Can you work these out from the model? Positions are in its coordinate system, mm. Face numbers are marked on the shaded views. A direction names the side the tool comes from. Round coordinates to 2 decimals unless told otherwise and drop trailing zeros. Loops run counter-clockwise (first coordinate to the right, second up) from the corner with the lowest first, then second, coordinate; pieces in that order, holes last. Notation, with made-up numbers: M 85,34.25 L 141,34.25 A20 cw 141,59.25 Z; hole C 59,25.25 d8. An arc over 180 degrees is marked long. Return JSON: item names as keys, results as strings.
Autodesk Fusion 360 part; units mm, degrees
sketch "Sketch1" plane through (0, 0, 0) normal (0, 1, 0) x (1, 0, 0)
  line L0 (0, 0) -> (12.5, 0)
  line L1 (12.5, 0) -> (12.5, -12.5)
  line L2 (12.5, -12.5) -> (0, -12.5)
  line L3 (0, -12.5) -> (0, 0)
  line L4 (11.25, -11.25) -> (1.25, -11.25)
  line L5 (1.25, -11.25) -> (1.25, -1.25)
  line L6 (1.25, -1.25) -> (11.25, -1.25)
  line L7 (11.25, -1.25) -> (11.25, -11.25)
  dimension "d1" = 12.5
  dimension "d2" = 90
  dimension "d3" = 12.5
  dimension "d4" = 1.25
extrude "Extrude1" add sketch "Sketch1" along normal blind 1 contours L4 L5 L6 L7
extrude "Extrude2" add sketch "Sketch1" along normal blind 45
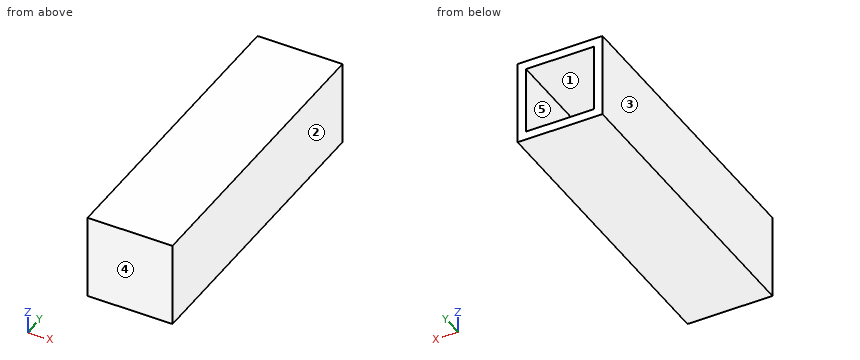
Q1. Suppose I cut it at A-A, the plane y = 16.5. Please give me the cut outline in (x, z), plus the area to 4 significant figures.
Results:
{"outline": "M 0,0 L 12.5,0 L 12.5,12.5 L 0,12.5 Z; hole M 1.25,1.25 L 11.25,1.25 L 11.25,11.25 L 1.25,11.25 Z", "area": "56.25 mm2"}
Q2. Suppose I cut it at B-B, the plane x = 9.25. Please give me the cut outline in (y, z).
Results:
{"outline": "M 0,0 L 45,0 L 45,1.25 L 1,1.25 L 1,11.25 L 45,11.25 L 45,12.5 L 0,12.5 Z"}
Q3. If I drill on line 1 along X through (y, z) = (25, 5.75); line 2 along Y through (x, z) = (6.25, 2), over which ranges is the centre line in solid material (lowest first)?
Results:
{"line 1": "x = 0 to 1.25, 11.25 to 12.5", "line 2": "y = 0 to 1"}
Q4. Suppose I cut it at C-C, the plane z = 8.5. Please give me the cut outline in (x, y), plus the area to 4 significant figures.
Results:
{"outline": "M 0,0 L 12.5,0 L 12.5,45 L 11.25,45 L 11.25,1 L 1.25,1 L 1.25,45 L 0,45 Z", "area": "122.5 mm2"}
Q5. Thinking about a two-plate mould opening in X: for the marked faces 1, 2 and 3, which applies, pulls with the +X half, pulls with the -X half, needs draft (parallel to the pull), parting line crosses it, or undercut?
Results:
{"face 1": "undercut", "face 2": "pulls with the +X half", "face 3": "pulls with the -X half"}
Q6. On a 3-axis mill with a long thin cutter (end or side, diameter ignored), from which of +Z, -Z, +X, -X, +Y, -Y can I reach the whole of each face in a straight line? I mean the marked faces 4 and 5. Say none if no direction works.
Results:
{"face 4": "+Z, -Z, +X, -X, -Y", "face 5": "+Y"}
